```python
from build123d import *

# Parameters (mm, degrees)
BOSS_EXTRUDE1_DEPTH = 60
SKETCH2_R           = 8.5
CUT_EXTRUDE1_DEPTH  = 108.703296143
FILLET1_R           = 2
SKETCH3_R           = 1
CUT_EXTRUDE2_DEPTH  = 10
SKETCH5_R           = 6.12
CUT_EXTRUDE3_DEPTH  = 3.58
SKETCH6_R           = 2.75
CUT_EXTRUDE4_DEPTH  = 107.030261718
CHAMFER1_SIZE       = 2
FILLET2_R           = 2


with BuildPart() as part:
    # Sketch1 → Boss-Extrude1 (new body)
    with BuildSketch(Plane(origin=(0, 0, 0), x_dir=(0, 0, -1), z_dir=(1, 0, 0))):
        Polygon((0, 0), (0, 80), (-20, 80), (-20, 20), (-60, 20), (-60, 0), align=None)
    extrude(amount=BOSS_EXTRUDE1_DEPTH)

    # Sketch2 → Cut-Extrude1 (cut, through all)
    with BuildSketch(Plane.XY.offset(20)):
        with Locations((30, 50)):
            Circle(SKETCH2_R)
    extrude(amount=-CUT_EXTRUDE1_DEPTH, mode=Mode.SUBTRACT)

    # Fillet1
    fillet1_edges = [part.edges().sort_by_distance(p)[0] for p in [
        (21.5, 50, 0),
        (21.5, 50, 20),
    ]]
    fillet(fillet1_edges, radius=FILLET1_R)

    # Sketch3 → Cut-Extrude2 (cut)
    with BuildSketch(Plane.XY.offset(20)):
        with Locations((10, 70.338969999)):
            Circle(SKETCH3_R)
        with Locations((50, 70.338969999)):
            Circle(SKETCH3_R)
        with Locations((50, 30.338969999)):
            Circle(SKETCH3_R)
        with Locations((10, 30.338969999)):
            Circle(SKETCH3_R)
    extrude(amount=-CUT_EXTRUDE2_DEPTH, mode=Mode.SUBTRACT)

    # Sketch5 → Cut-Extrude3 (cut)
    with BuildSketch(Plane(origin=(0, 20, 0), x_dir=(1, 0, 0), z_dir=(0, 1, 0))):
        with Locations(Location((45, -50, 0), (0, 0, 270))):
            Circle(SKETCH5_R)
    extrude(amount=-CUT_EXTRUDE3_DEPTH, mode=Mode.SUBTRACT)

    # Sketch6 → Cut-Extrude4 (cut, through all)
    with BuildSketch(Plane(origin=(0, 16.42, 0), x_dir=(1, 0, 0), z_dir=(0, 1, 0))):
        with Locations(Location((45, -50, 0), (0, 0, 270))):
            Circle(SKETCH6_R)
    extrude(amount=-CUT_EXTRUDE4_DEPTH, mode=Mode.SUBTRACT)

    # Chamfer1
    chamfer1_edges = [part.edges().sort_by_distance(p)[0] for p in [
        (30, 20, 60),
        (60, 20, 40),
        (0, 20, 40),
    ]]
    chamfer(chamfer1_edges, length=CHAMFER1_SIZE)

    # Fillet2
    fillet2_edges = [part.edges().sort_by_distance(p)[0] for p in [
        (30, 20, 20),
    ]]
    fillet(fillet2_edges, radius=FILLET2_R)


solid = part.part
```
Can you work these out from the model? Positions are in its coordinate system, mm. A direction names the side the tool comes from. Give positions to 0.01 mm unless a question says otherwise; leave off trailing zeros. Loops run counter-clockwise (first coordinate to the right, second up) from the corner with the lowest first, then second, coordinate; pieces in that order, holes last. Notation, with made-up numbers: M 30,18 L 51,18 A14 cw 51,39 Z; hole C 80,32.25 d2. An arc over 180 degrees is marked long. Answer in a Markdown table with one row per item.
1. If I drill on line 1 along Y through (x, z) = (50, 16); line 2 along X through (y, z) = (49, 18.5); line 3 along Y through (x, z) = (55, 34.5), over which ranges is the centre line in solid material (lowest first)?
Taken from the geometry:
| item | result |
|---|---|
| line 1 | y = 0 to 29.34, 31.34 to 69.34, 71.34 to 80 |
| line 2 | x = 0 to 21.5, 38.5 to 60 |
| line 3 | y = 0 to 20 |
2. Which directions (+Z, -Z, +X, -X, +Y, -Y) give clear straight access to the entire face, cutting with the end or side of a thin tool? Please do faces 4 (the cylindrical face through (50.924, 29.956, 15.07)), 5 (the flat face through (59, 19, 40)), 6 (the flat face through (42, 16.42, 51)), 7 (the flat face through (0, 32, 17)).
Taken from the geometry:
| item | result |
|---|---|
| face 4 | +Z |
| face 5 | +Z, +X, +Y |
| face 6 | +Y |
| face 7 | +Z, -Z, -X, +Y, -Y |
3. Suppose I cut it at B-B on z = 50. Write out the boundary of the cut face in (x, y), plus the area to 3 significant figures.
Taken from the geometry:
| item | result |
|---|---|
| outline | M 0,0 L 42.25,0 L 42.25,16.42 L 38.88,16.42 L 38.88,20 L 2,20 L 0,18 Z; M 47.75,0 L 60,0 L 60,18 L 58,20 L 51.12,20 L 51.12,16.42 L 47.75,16.42 Z |
| area | 1,060 mm² |
4. Suppose I cut it at A-A on x = 45. Write out the boundary of the cut face in (y, z), plus the area to 3 significant figures.
Taken from the geometry:
| item | result |
|---|---|
| outline | M 0,0 L 80,0 L 80,20 L 22,20 A2 cw 20,22 L 20,43.88 L 16.42,43.88 L 16.42,47.25 L 0,47.25 Z; M 0,52.75 L 16.42,52.75 L 16.42,56.12 L 20,56.12 L 20,58 L 18,60 L 0,60 Z |
| area | 2,260 mm² |
5. Suppose I cut it at C-C on x = 10. Write out the boundary of the cut face in (y, z).
Taken from the geometry:
| item | result |
|---|---|
| outline | M 0,0 L 80,0 L 80,20 L 71.34,20 L 71.34,10 L 69.34,10 L 69.34,20 L 31.34,20 L 31.34,10 L 29.34,10 L 29.34,20 L 22,20 A2 cw 20,22 L 20,58 L 18,60 L 0,60 Z |
6. Thinking about a two-plate mould opening in X: for faces 1 (the flat face through (30, 0, 30)), 2 (the cylindrical face through (9.87, 71.33, 15.07)), 3 (the flat face through (1, 19, 40)), which applies, released by +X, released by -X, zero draft, split by the parting line, or undercut?
Taken from the geometry:
| item | result |
|---|---|
| face 1 | zero draft |
| face 2 | undercut |
| face 3 | released by -X |
7. Suppose I cut it at D-D on z = 12. Write out the boundary of the cut face in (x, y).
Taken from the geometry:
| item | result |
|---|---|
| outline | M 0,0 L 60,0 L 60,80 L 0,80 Z; hole C 10,30.34 d2; hole C 10,70.34 d2; hole C 30,50 d17; hole C 50,30.34 d2; hole C 50,70.34 d2 |
8. For pin 1 Ø13.5 at (x, z) = (42.5, 51.5) entering from +Y; pin 2 Ø1.2 at (x, y) = (50, 30.34) entering from +Z; pin 3 Ø2.5 at (x, y) = (10, 30.34) entering from +Z; pin 4 Ø10 at (x, y) = (30, 50) entering from +Z, each with a flat end and sliding along its axis, tell me the tip position at first contact or that it passes through.
Taken from the geometry:
| item | result |
|---|---|
| pin 1 | stops at y = 20 |
| pin 2 | stops at z = 10 |
| pin 3 | stops at z = 20 |
| pin 4 | passes through |
